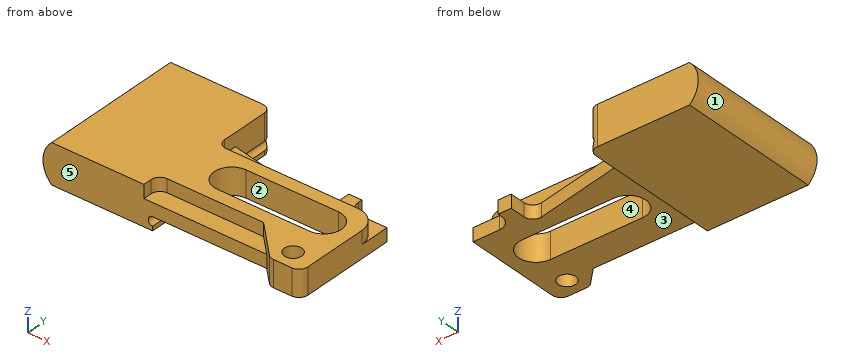
```python
from build123d import *

# Parameters (mm, degrees)
EXTRUSION1_DEPTH        = 6
NERVURE1_REACH          = 70.739
ESQUISSE2_WALL_W        = 167.477270848
ESQUISSE2_WALL_H        = 3
ENL_V_MAT_EXTRU_1_DEPTH = 69.738635424
NERVURE2_REACH          = 70.739
ESQUISSE4_WALL_W        = 164.972368416
ESQUISSE4_WALL_H        = 3
CONG_1_R                = 2
CONG_3_R                = 5
NERVURE4_START          = -3
NERVURE4_DEPTH          = 3
CONG_4_R                = 3
CONG_5_R                = 2
ESQUISSE6_W             = 23
ESQUISSE6_H             = 33
EXTRUSION2_DEPTH        = 3
EXTRUSION3_DEPTH        = 33
CONG_7_R                = 2
ESQUISSE9_R             = 1
ENL_V_MAT_EXTRU_2_DEPTH = 71.746024717
ESQUISSE10_R            = 2
ENL_V_MAT_EXTRU_3_DEPTH = 70.065186747


# Read off the part's stored shape, not the designer's step: Nervure4
with BuildPart() as part:
    # Esquisse1 → Extrusion1 (new body)
    with BuildSketch(Plane.XY):
        Polygon((0, 0), (0, 33), (23, 33), (23, 18), (60, 18), (60, -4), (53, -4), (45, 4), (21, 4), (21, 0), align=None)
    extrude(amount=EXTRUSION1_DEPTH)

    # Esquisse2 wall → Nervure1 (add, up to next)
    with BuildSketch(Plane(origin=(35, 0, 0), x_dir=(1, 0, 0), z_dir=(0, -1, 0)), mode=Mode.PRIVATE) as nervure1_sk1:
        with Locations((0, 1.5)):
            Rectangle(ESQUISSE2_WALL_W, ESQUISSE2_WALL_H)
    nervure1_tool1 = extrude(nervure1_sk1.sketch, amount=-NERVURE1_REACH, mode=Mode.PRIVATE) - part.part
    add(nervure1_tool1.solids().sort_by_distance((35, 0, 0))[0])

    # Esquisse3 → Enlèv. mat.-Extru.1 (cut, through all)
    with BuildSketch(Plane.XY.offset(6)):
        with BuildLine():
            Line((32, 15), (53, 15))
            ThreePointArc((53, 15), (57, 11), (53, 7))
            Line((53, 7), (32, 7))
            ThreePointArc((32, 7), (28, 11), (32, 15))
        make_face()
    extrude(amount=-ENL_V_MAT_EXTRU_1_DEPTH, mode=Mode.SUBTRACT)

    # Esquisse4 wall → Nervure2 (add, up to next)
    with BuildSketch(Plane(origin=(35.5, 20.5, 0), x_dir=(0.980580675691, -0.196116135138, 0), z_dir=(-0.196116135138, -0.980580675691, 0)), mode=Mode.PRIVATE) as nervure2_sk1:
        with Locations((0, 1.5)):
            Rectangle(ESQUISSE4_WALL_W, ESQUISSE4_WALL_H)
    nervure2_tool1 = extrude(nervure2_sk1.sketch, amount=NERVURE2_REACH, mode=Mode.PRIVATE) - part.part
    add(nervure2_tool1.solids().sort_by_distance((35.5, 20.5, 0))[0])

    # Congé1
    cong_1_edges = [part.edges().sort_by_distance(p)[0] for p in [
        (23, 18, 4.5),
        (21, 4, 4.5),
    ]]
    fillet(cong_1_edges, radius=CONG_1_R)

    # Congé3
    cong_3_edges = [part.edges().sort_by_distance(p)[0] for p in [
        (60, 18, 3),
    ]]
    fillet(cong_3_edges, radius=CONG_3_R)

    # Nervure4 outline → Nervure4 (add)
    with BuildSketch(Plane(origin=(0, 0, 0), x_dir=(-1, 0, 0), z_dir=(0, 0, -1)).offset(NERVURE4_START)):
        with BuildLine():
            Line((-60, 20), (-60, 13))
            ThreePointArc((-60, 13), (-58.535533906, 16.535533906), (-55, 18))
            Line((-55, 18), (-48, 18))
            Line((-48, 18), (-48, 24))
            Line((-48, 24), (-51, 24))
            Line((-51, 24), (-51, 20))
            Line((-51, 20), (-60, 20))
        make_face()
    extrude(amount=NERVURE4_DEPTH)

    # Congé4
    cong_4_edges = [part.edges().sort_by_distance(p)[0] for p in [
        (51, 20, 1.5),
    ]]
    fillet(cong_4_edges, radius=CONG_4_R)

    # Congé5
    cong_5_edges = [part.edges().sort_by_distance(p)[0] for p in [
        (48, 18, 1.5),
    ]]
    fillet(cong_5_edges, radius=CONG_5_R)

    # Esquisse6 → Extrusion2 (add)
    with BuildSketch(Plane(origin=(0, 0, 0), x_dir=(-1, 0, 0), z_dir=(0, 0, -1))):
        with Locations((-11.5, 16.5)):
            Rectangle(ESQUISSE6_W, ESQUISSE6_H)
    extrude(amount=EXTRUSION2_DEPTH)

    # Esquisse8 → Extrusion3 (add)
    with BuildSketch(Plane(origin=(0, 33, 0), x_dir=(1, 0, 0), z_dir=(0, 1, 0))):
        with BuildLine():
            Line((0, 3), (0, -6))
            ThreePointArc((0, -6), (-2, -1.5), (0, 3))
        make_face()
    extrude(amount=-EXTRUSION3_DEPTH)

    # Congé7
    cong_7_edges = [part.edges().sort_by_distance(p)[0] for p in [
        (23, 33, 1.5),
        (60, -4, 3),
        (53, -4, 3),
    ]]
    fillet(cong_7_edges, radius=CONG_7_R)

    # Esquisse9 → Enlèv. mat.-Extru.2 (cut, through all)
    with BuildSketch(Plane(origin=(0, 33, 0), x_dir=(1, 0, 0), z_dir=(0, 1, 0))):
        with Locations((23, 1)):
            Circle(ESQUISSE9_R)
    extrude(amount=-ENL_V_MAT_EXTRU_2_DEPTH, mode=Mode.SUBTRACT)

    # Esquisse10 → Enlèv. mat.-Extru.3 (cut, through all)
    with BuildSketch(Plane.XY.offset(6)):
        with Locations((55, 0)):
            Circle(ESQUISSE10_R)
    extrude(amount=-ENL_V_MAT_EXTRU_3_DEPTH, mode=Mode.SUBTRACT)


solid = part.part
```
The model under review builds one solid part; all positions refer to its coordinate system, in mm. Face numbers are marked on the shaded views. A direction names the side the tool comes from. Round coordinates to 2 decimals unless told otherwise and drop trailing zeros. Loops run counter-clockwise (first coordinate to the right, second up) from the corner with the lowest first, then second, coordinate; pieces in that order, holes last.
1) Tool access review of the marked faces 1 and 2: name each direction out of +Z, -Z, +X, -X, +Y, -Y from which nothing blocks a thin tool from reaching the whole face with its end or side.
Values follow:
face 1: -X, +Y, -Y
face 2: +Z, -Z
2) Wall thickness on line 1 along Y through (x, z) = (55, 3.15); line 2 along Y through (x, z) = (55, 1.5); line 3 along Z through (x, y) = (51.5, 0): over which ranges is each line inside the solid? List them lowest first.
Values follow:
line 1: y = -4 to -2, 2 to 7.54, 14.46 to 18
line 2: y = -4 to -2, 2 to 7.54, 14.46 to 20
line 3: z = 0 to 6
3) Consider section C-C on z = 1.5. State the section outline as (x, y) points.
Values follow:
outline: (-2, 0) - (49, 0) - (52.41, -3.41) arc R2 ccw to (53.83, -4) - (58, -4) arc R2 ccw to (60, -2) - (60, 20) - (54, 20) arc R3 cw to (51, 23) - (51, 24) - (48, 24) - (48, 20.44) arc R2 cw to (45.61, 18.48) - (23, 23) - (23, 31) arc R2 ccw to (21, 33) - (-2, 33) - close; hole (32, 7) - (53, 7) arc R4 ccw to (53, 15) - (32, 15) arc R4 ccw to start; hole circle Ø4 at (55, 0)
4) Consider section A-A on x = 39. State the section outline as (y, z) points, then the cut area to 3 significant figures.
Values follow:
outline: (0, 0) - (7, 0) - (7, 6) - (4, 6) - (4, 3) - (0, 3) - close; (15, 0) - (19.8, 0) - (19.8, 3) - (18, 3) - (18, 6) - (15, 6) - close
area: 53.4 mm2
5) The part is to be moulded in two halves that separate along Y. For the marked faces 3, 4 and 5, say which applies: pulls with the +Y half, pulls with the -Y half, needs draft (parallel to the pull), parting line crosses it, or undercut.
Values follow:
face 3: needs draft
face 4: undercut
face 5: pulls with the -Y half
6) Clearance check with flat-ended pins moving along their axes: P1, Ø2, axis at x = 25, y = 26, coming from the -Z side; P2, Ø5, axis at x = 6, z = 4.5, coming from the -Y side; P3, Ø1.5, axis at x = 34.5, z = 4, coming from the -Y side; P4, Ø1, axis at y = 4.5, z = 4, coming from the -X side. State where each tip first meets the part, or that it passes through.
Values follow:
P1: passes through
P2: stops at y = 0
P3: stops at y = 4
P4: stops at x = -1.66
7) Consider section D-D on y = 26. State the section outline as (x, z) points (1 decimal).
Values follow:
outline: (0, -3) - (23, -3) - (23, -2) arc R1 cw to (23, 0) - (23, 6) - (0, 6) arc R6.1 ccw to start
8) Consider section B-B on y = 11. State the section outline as (x, z) points (1 decimal), then the cut area to 3 significant figures.
Values follow:
outline: (0, -3) - (23, -3) - (23, -2) arc R1 cw to (23, 0) - (28, 0) - (28, 6) - (0, 6) arc R6.1 ccw to start; (57, 0) - (60, 0) - (60, 6) - (57, 6) - close
area: 266 mm2
